Here's how the part is built. I have some questions about the finished solid (model axes, mm). A direction names the side the tool comes from. Coordinates: 2 decimals unless noted, no trailing zeros. Order: outer loops, then holes, each group sorted by start corner. A loop starts at its lowest first (then second) coordinate and runs counter-clockwise, first axis right, second up. Notation, with made-up numbers: (0.5, 73) - (46.5, 73) arc R24 cw to (46.5, 104) - close; hole circle Ø4 at (-38, 3.25). An arc over 180 degrees is marked (long way). Answer as CSV lines item,"result". Start each with the question number.
Item 1: We'd pull the mould along Y, two halves only. Please class faces 6 (the face through (46, 17.75, 28)), 7 (the face through (-48, 15.75, 25)), 8 (the face through (15, -6, 9)): pulls with the +Y half, pulls with the -Y half, needs draft (parallel to the pull), parting line crosses it, or undercut.
Item 2: Imagine slicing it at D-D on z = -23.5. List the corners of the cut face in (x, y) for me, and give its area (3 significant figures).
Item 3: Imagine slicing it at B-B on x = 26. List the corners of the cut face in (y, z) for me.
Item 4: Imagine slicing it at A-A on z = -9.75. List the corners of the cut face in (x, y) for me, and give its area (3 significant figures).
Item 5: I'm going to push flat-ended pins straight in: pin 1 (4.5 mm diameter, centred on x = -36, z = 25.5, fed in from +Y); pin 2 (8 mm diameter, centred on y = 21, z = 6.5, fed in from -X); pin 3 (0.9 mm diameter, centred on x = 41, z = 21, fed in from -Y); pin 4 (3 mm diameter, centred on x = 5.65, z = -9.75, fed in from -Y). Where does each tip first touch, or does it pass through?
Item 6: I need wall thicknesses on line 1 (Y direction, x = 5.65, z = 4.5); line 2 (X direction, y = -24.2, z = 32.75); line 3 (Z direction, x = 56, y = 5). Which ranges of each line are inside material? Lowest first, please.
Item 7: Imagine slicing it at C-C on y = -9.5. List the corners of the cut face in (x, z) for me, and give its area (4 significant figures).
Item 8: On a 3-axis mill with a long thin cutter (end or side, diameter ignored), from which of +Z, -Z, +X, -X, +Y, -Y can I reach the whole of each face in a straight line? I mean faces 1 (the face through (-10.35, 0, 20)), 2 (the face through (-48, 4.75, 25)), 3 (the face through (6, -24, 0)), 4 (the face through (0, -23, -63.75)), 5 (the face through (-9.15, 24, 18)). Say none if no direction works.
from build123d import *

# Parameters (mm, degrees)
SKETCH1_W           = 30
SKETCH1_H           = 55
SKETCH1_R           = 1.55
SKETCH1_W_2         = 20.7
SKETCH1_H_2         = 40.5
BOSS_EXTRUDE1_DEPTH = 35
SKETCH11_W          = 30
SKETCH11_H          = 7.25
BOSS_EXTRUDE5_DEPTH = 63.75
SKETCH12_R          = 1.55
CUT_EXTRUDE2_DEPTH  = 13
LPATTERN2_COUNT     = 2
LPATTERN2_PITCH     = 48
FILLET1_R           = 4
SKETCH13_W          = 60
SKETCH13_H          = 15
BOSS_EXTRUDE6_DEPTH = 15
CUT_EXTRUDE3_DEPTH  = 55
CUT_EXTRUDE4_DEPTH  = 55
SKETCH18_W          = 18.3
SKETCH18_H          = 21
CUT_EXTRUDE5_DEPTH  = 113.756651688
FILLET6_R           = 2
FILLET7_R           = 2
FILLET8_R           = 2


with BuildPart() as part:
    # Sketch1 → Boss-Extrude1 (new body)
    with BuildSketch(Plane.XY):
        Rectangle(SKETCH1_W, SKETCH1_H)
        with Locations((5.65, 24.2)):
            Circle(SKETCH1_R, mode=Mode.SUBTRACT)
        with Locations(Location((-5.65, 24.2, 0), (0, 0, 180))):
            Circle(SKETCH1_R, mode=Mode.SUBTRACT)
        with Locations((-5.65, -24.2)):
            Circle(SKETCH1_R, mode=Mode.SUBTRACT)
        with Locations(Location((5.65, -24.2, 0), (0, 0, 180))):
            Circle(SKETCH1_R, mode=Mode.SUBTRACT)
        Rectangle(SKETCH1_W_2, SKETCH1_H_2, mode=Mode.SUBTRACT)
    extrude(amount=BOSS_EXTRUDE1_DEPTH)

    # Sketch11 → Boss-Extrude5 (add)
    with BuildSketch(Plane(origin=(0, 0, 0), x_dir=(-1, 0, 0), z_dir=(0, 0, -1))):
        with Locations((0, -23.875)):
            Rectangle(SKETCH11_W, SKETCH11_H)
    extrude(amount=BOSS_EXTRUDE5_DEPTH)

    # Sketch12 → Cut-Extrude2 (cut)
    with BuildSketch(Plane.XZ.offset(27.5)):
        with Locations(Location((-5.65, -57.75, 0), (0, 0, 270))):
            Circle(SKETCH12_R)
        with Locations(Location((5.65, -57.75, 0), (0, 0, 270))):
            Circle(SKETCH12_R)
    cut_extrude2 = extrude(amount=-CUT_EXTRUDE2_DEPTH, mode=Mode.SUBTRACT)

    # LPattern2: Cut-Extrude2 ×2
    with Locations(*[(0, 0, i * LPATTERN2_PITCH) for i in range(1, LPATTERN2_COUNT)]):
        add(cut_extrude2, mode=Mode.SUBTRACT)

    # Fillet1
    fillet1_edges = [part.edges().sort_by_distance(p)[0] for p in [
        (12.675, -20.25, 0),
        (-12.675, -20.25, 0),
        (15, -23.875, -63.75),
        (-15, -23.875, -63.75),
    ]]
    fillet(fillet1_edges, radius=FILLET1_R)

    # Sketch13 → Boss-Extrude6 (add)
    with BuildSketch(Plane.XY.offset(35)):
        with Locations((-45, 10.25)):
            Rectangle(SKETCH13_W, SKETCH13_H)
        with Locations((45, 10.25)):
            Rectangle(SKETCH13_W, SKETCH13_H)
    extrude(amount=-BOSS_EXTRUDE6_DEPTH)

    # Sketch14 → Cut-Extrude3 (cut)
    with BuildSketch(Plane(origin=(75, 0, 0), x_dir=(0, 0, -1), z_dir=(1, 0, 0))):
        Polygon((-35, 13.25), (-35, 7.25), (-27, 7.25), (-27, 4.75), (-23, 4.75), (-23, 7.25), (-20, 7.25), (-20, 13.25), (-23, 13.25), (-23, 15.75), (-27, 15.75), (-27, 13.25), align=None)
    extrude(amount=-CUT_EXTRUDE3_DEPTH, mode=Mode.SUBTRACT)

    # Sketch17 → Cut-Extrude4 (cut)
    with BuildSketch(Plane.ZY.offset(75)):
        Polygon((35, 7.25), (35, 13.25), (27, 13.25), (27, 15.75), (23, 15.75), (23, 13.25), (20, 13.25), (20, 7.25), (23, 7.25), (23, 4.75), (27, 4.75), (27, 7.25), align=None)
    extrude(amount=-CUT_EXTRUDE4_DEPTH, mode=Mode.SUBTRACT)

    # Sketch18 → Cut-Extrude5 (cut, through all)
    with BuildSketch(Plane(origin=(0, 27.5, 0), x_dir=(1, 0, 0), z_dir=(0, 1, 0))):
        with Locations((0, -17.5)):
            Rectangle(SKETCH18_W, SKETCH18_H)
    extrude(amount=-CUT_EXTRUDE5_DEPTH, mode=Mode.SUBTRACT)

    # Fillet6
    # the kernel refuses this fillet: 2 mm, written as the material it adds along each edge
    with BuildSketch(Plane(origin=(-15, 17.75, 35), x_dir=(0, 1, 0), z_dir=(0, 0, -1))) as fillet6_piece_1:
        with BuildLine():
            CenterArc((FILLET6_R, -FILLET6_R), FILLET6_R, 90, 90)
            Line((0, -FILLET6_R), (0, 0))
            Line((0, 0), (FILLET6_R, 0))
        make_face()
    extrude(amount=15)
    with BuildSketch(Plane(origin=(15, 17.75, 35), x_dir=(0, 1, 0), z_dir=(0, 0, -1))) as fillet6_piece_2:
        with BuildLine():
            CenterArc((FILLET6_R, FILLET6_R), FILLET6_R, 180, 90)
            Line((0, FILLET6_R), (0, 0))
            Line((0, 0), (FILLET6_R, 0))
        make_face()
    extrude(amount=15)
    # the kernel refuses this fillet: 2 mm, written as the material it takes off along each edge
    with BuildSketch(Plane(origin=(-20, 27.5, 0), x_dir=(0, 0, 1), z_dir=(1, 0, 0))) as fillet6_2_piece_1:
        with BuildLine():
            CenterArc((FILLET6_R, FILLET6_R), FILLET6_R, 180, 90)
            Line((0, FILLET6_R), (0, 0))
            Line((0, 0), (FILLET6_R, 0))
        make_face()
    extrude(amount=40, mode=Mode.SUBTRACT)
    with BuildSketch(Plane(origin=(-15, 27.5, -5), x_dir=(0, -1, 0), z_dir=(0, 0, 1)), Plane(origin=(15, 27.5, -5), x_dir=(-1, 0, 0), z_dir=(0, 0, 1))) as fillet6_2_piece_2:
        with BuildLine():
            CenterArc((FILLET6_R, FILLET6_R), FILLET6_R, 180, 90)
            Line((0, FILLET6_R), (0, 0))
            Line((0, 0), (FILLET6_R, 0))
        make_face()
    extrude(amount=45, mode=Mode.SUBTRACT)
    with BuildSketch(Plane(origin=(-20, 27.5, 35), x_dir=(0, 0, -1), z_dir=(1, 0, 0))) as fillet6_2_piece_3:
        with BuildLine():
            CenterArc((FILLET6_R, -FILLET6_R), FILLET6_R, 90, 90)
            Line((0, -FILLET6_R), (0, 0))
            Line((0, 0), (FILLET6_R, 0))
        make_face()
    extrude(amount=40, mode=Mode.SUBTRACT)

    # Fillet7
    fillet7_edges = [part.edges().sort_by_distance(p)[0] for p in [
        (-15, 2.75, 27.5),
        (15, 2.75, 27.5),
    ]]
    fillet(fillet7_edges, radius=FILLET7_R)

    # Fillet8
    fillet8_edges = [part.edges().sort_by_distance(p)[0] for p in [
        (15, -27.5, -12.375),
        (-15, -27.5, -12.375),
        (0, -27.5, -63.75),
        (-13.828427125, -27.5, -62.578427125),
        (13.828427125, -27.5, -62.578427125),
    ]]
    fillet(fillet8_edges, radius=FILLET8_R)


solid = part.part
Responses:
1,face 6,"pulls with the +Y half"
1,face 7,"undercut"
1,face 8,"needs draft"
2,outline,"(-15, -25.5) arc R2 ccw to (-13, -27.5) - (13, -27.5) arc R2 ccw to (15, -25.5) - (15, -20.25) - (-15, -20.25) - close"
2,area,"216 mm^2"
3,outline,"(2.75, 20) - (7.25, 20) - (7.25, 23) - (4.75, 23) - (4.75, 27) - (7.25, 27) - (7.25, 35) - (2.75, 35) - close; (13.25, 20) - (17.75, 20) - (17.75, 35) - (13.25, 35) - (13.25, 27) - (15.75, 27) - (15.75, 23) - (13.25, 23) - close"
4,outline,"(-15, -25.5) arc R2 ccw to (-13, -27.5) - (-7.2, -27.5) - (-7.2, -20.25) - (-15, -20.25) - close; (-4.1, -27.5) - (4.1, -27.5) - (4.1, -20.25) - (-4.1, -20.25) - close; (7.2, -27.5) - (13, -27.5) arc R2 ccw to (15, -25.5) - (15, -20.25) - (7.2, -20.25) - close"
4,area,"171 mm^2"
5,pin 1,"stops at y = 17.75"
5,pin 2,"stops at x = -15"
5,pin 3,"stops at y = 2.75"
5,pin 4,"passes through"
6,line 1,"y = -27.5 to -25.75, -22.65 to -20.25, 20.25 to 22.65, 25.75 to 27.5"
6,line 2,"x = -15 to -7.2, -4.1 to 4.1, 7.2 to 15"
6,line 3,"z = 20 to 23, 27 to 35"
7,outline,"(-15, 0) - (-10.35, 0) - (-10.35, 35) - (-15, 35) - close; (10.35, 0) - (15, 0) - (15, 35) - (10.35, 35) - close"
7,area,"325.5 mm^2"
8,face 1,"+Z, -Z"
8,face 2,"-X"
8,face 3,"+Z"
8,face 4,"-Z, +X, -X, +Y, -Y"
8,face 5,"+Y, -Y"
